Part print with two shaded views. Sizes in mm from the minimum x, y, z corner. A direction names the side the tool comes from. Round coordinates to 2 decimals unless told otherwise and drop trailing zeros. Write each loop counter-clockwise with the first axis right and the second up, starting at its lowest first coordinate (ties: lowest second). Pieces come first, ordered by that corner, then holes. Notation, with made-up numbers: (74.5, -24) -> (105.5, -24) arc R31 ccw to (105.5, 15) -> close; hole circle Ø6 at (3, -32). An arc over 180 degrees is marked (long way). Put each result on its own line as item: value. Start each with the question number.
1. Saw through at A-A on z = 17. List the corners of the cut face in (x, y), and give its area (3 significant figures).
2. Saw through at C-C on x = 128. List the corners of the cut face in (y, z) (3 decimals), and give its area (3 significant figures).
3. Flat gauge pins, fed straight in: P1, Ø21.5, axis at x = 121, z = 42.5, coming from the +Y side; P2, Ø22.5, axis at y = 33.5, z = 86.5, coming from the +X side; P3, Ø10, axis at x = 151, z = 61, coming from the +Y side. Where does each tip first touch, or does it go through?
4. Drill centre lines: line 1 (Y direction, x = 152.5, z = 127); line 2 (X direction, y = 65, z = 37); line 3 (Y direction, x = 121, z = 86.5). Where is each one in solid material? Low to high. Write a range as from..to.
5. Saw through at B-B on y = 20. List the corners of the cut face in (x, z) (3 decimals), and give its area (3 significant figures).
6. 3-axis set-ups, long thin cutter, end or side, ignore diameter. For the marked faces 1 and 2: which of +Z, -Z, +X, -X, +Y, -Y reach the whole face in a straight line?
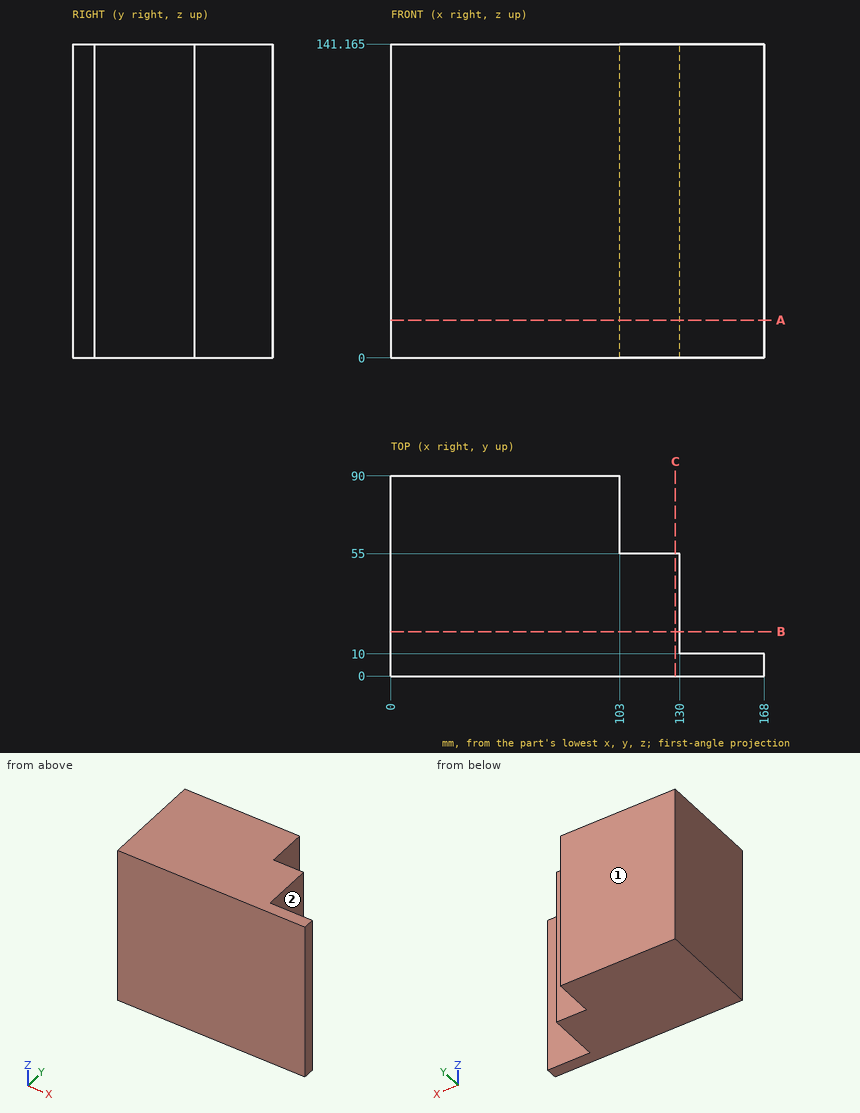
Return value:
1. outline: (0, 0) -> (168, 0) -> (168, 10) -> (130, 10) -> (130, 55) -> (103, 55) -> (103, 90) -> (0, 90) -> close
1. area: 11,100 mm^2
2. outline: (0, 0) -> (55, 0) -> (55, 141.165) -> (0, 141.165) -> close
2. area: 7,760 mm^2
3. P1: stops at y = 55
3. P2: stops at x = 130
3. P3: stops at y = 10
4. line 1: y = 0..10
4. line 2: x = 0..103
4. line 3: y = 0..55
5. outline: (0, 0) -> (130, 0) -> (130, 141.165) -> (0, 141.165) -> close
5. area: 18,400 mm^2
6. face 1: +Z, -Z, +X, -X, +Y
6. face 2: +Z, -Z, +X, +Y
